Could you check a few things on this model? Use its own coordinates, in mm. A direction names the side the tool comes from. Give positions to 0.01 mm unless a question says otherwise; leave off trailing zeros. Write each loop counter-clockwise with the first axis right and the second up, starting at its lowest first coordinate (ties: lowest second). Pieces come first, ordered by that corner, then holes. Notation, with made-up numbers: M 50,47 L 94,47 A21 ccw 94,75 Z; hole C 23.25,-14.75 d3. An arc over 180 degrees is marked long. One line per item, written item: value.
```python
from build123d import *

# Parameters (mm, degrees)
F0_W     = 2
F0_H     = 7
F0_W_2   = 3
F0_H_2   = 12
F1_DEPTH = 7
F2_R     = 1.5
F3_DEPTH = 12
F4_R     = 3
F5_R     = 1.5
F6_DEPTH = 25
F7_R     = 1


with BuildPart() as f1:
    # F0 (on Top) → F1 (new body)
    with BuildSketch(Plane.XY):
        with Locations((-3, -4.5)):
            Rectangle(F0_W, F0_H)
        with Locations((-6, 7)):
            Rectangle(F0_W_2, F0_H_2)
        with Locations((6, 7)):
            Rectangle(F0_W_2, F0_H_2)
        Polygon((4, -1), (7.5, -1), (7.5, 1), (4.5, 1), (-4.5, 1), (-7.5, 1), (-7.5, -1), (-4, -1), (-2, -1), (2, -1), align=None)
        with Locations((3, -4.5)):
            Rectangle(F0_W, F0_H)
    extrude(amount=F1_DEPTH)

    # F2 (on face) → F3 (cut)
    with BuildSketch(Plane.YZ.offset(4)):
        with Locations((-4.5, 3.5)):
            Circle(F2_R)
    extrude(amount=-F3_DEPTH, mode=Mode.SUBTRACT)

    # F4
    f4_edges = [f1.edges().sort_by_distance(p)[0] for p in [
        (-3, -8, 0),
        (3, -8, 0),
        (3, -8, 7),
        (-3, -8, 7),
        (-6, 13, 0),
        (6, 13, 0),
        (-6, 13, 7),
        (6, 13, 7),
    ]]
    fillet(f4_edges, radius=F4_R)

    # F5 (on face) → F6 (cut)
    with BuildSketch(Plane(origin=(-7.5, 0, 0), x_dir=(0, -1, 0), z_dir=(-1, 0, 0))):
        with Locations((-9.5, 3.5)):
            Circle(F5_R)
    extrude(amount=-F6_DEPTH, mode=Mode.SUBTRACT)

    # F7
    f7_edges = [f1.edges().sort_by_distance(p)[0] for p in [
        (4.5, 11, 3.5),
        (-4.5, 11, 3.5),
    ]]
    fillet(f7_edges, radius=F7_R)


solid = f1.part
```
1) I'm going to push flat-ended pins straight in: pin 1 (1.8 mm diameter, centred on x = 5.5, z = 2, fed in from -Y); pin 2 (2 mm diameter, centred on x = 0.5, z = 4.5, fed in from +Y); pin 3 (3 mm diameter, centred on x = -5, z = 2, fed in from -Y); pin 4 (2 mm diameter, centred on y = -6, z = 4, fed in from +X). Where does each tip first touch, or does it pass through?
Outcome:
pin 1: stops at y = -1
pin 2: stops at y = 1
pin 3: stops at y = -8
pin 4: stops at x = 4
2) If we section it at A-A, the plane y = 5.25: Write out the boundary of the cut face in (x, z), then the cut area to 3 significant figures.
Outcome:
outline: M -7.5,0 L -4.5,0 L -4.5,7 L -7.5,7 Z; M 4.5,0 L 7.5,0 L 7.5,7 L 4.5,7 Z
area: 42.0 mm^2
3) If we section it at D-D, the plane z = 3.5: Give the number of separate pieces and of enclosed holes in the cut face, then the cut area to 3 significant figures.
Outcome:
separate pieces: 5
enclosed holes: 0
area: 99.1 mm^2
4) On a 3-axis mill with a long thin cutter (end or side, diameter ignored), from which of +Z, -Z, +X, -X, +Y, -Y can I reach the whole of each face in a straight line? I mean faces 5 (the face through (6, -1, 3)), 6 (the face through (3, -8, 3.5)), 7 (the face through (0, 1, 3)), 8 (the face through (-6, -1, 3)), 9 (the face through (2, -3, 4.2)). Say none if no direction works.
Outcome:
face 5: +Z, -Z, +X, -Y
face 6: +Z, -Z, +X, -X, -Y
face 7: +Z, -Z, +Y
face 8: +Z, -Z, -X, -Y
face 9: +Z, -Z, -Y
5) Please list where these lines run through material, in increasing order: L1, parallel to Z at x = -6.8, y = 9.5; L2, parallel to X at y = 4, z = 3; L3, parallel to Y at x = 5.5, z = 4.75. Write a range as from..to.
Outcome:
L1: z = 0..2, 5..7
L2: x = -7.5..-4.5, 4.5..7.5
L3: y = -1..8.67, 10.33..12.9
6) If we section it at C-C, the plane x = -6: Write out the boundary of the cut face in (y, z).
Outcome:
outline: M -1,0 L 10,0 A3 ccw 13,3 L 13,4 A3 ccw 10,7 L -1,7 Z; hole C 9.5,3.5 d3
7) If we section it at B-B, the plane y = 9.5: Write out the boundary of the cut face in (x, z), then the cut area to 3 significant figures.
Outcome:
outline: M -7.5,0 L -4.5,0 L -4.5,1 A1 ccw -5.5,2 L -7.5,2 Z; M -7.5,5 L -5.5,5 A1 ccw -4.5,6 L -4.5,7 L -7.5,7 Z; M 4.5,0 L 7.5,0 L 7.5,2 L 5.5,2 A1 ccw 4.5,1 Z; M 4.5,6 A1 ccw 5.5,5 L 7.5,5 L 7.5,7 L 4.5,7 Z
area: 23.1 mm^2
8) We'd pull the mould along X, two halves only. Please class faces 1 (the face through (-2, -3, 4.2)), 2 (the face through (-4, -3, 4.2)), 3 (the face through (6.02, 12.1, 6.14)), 4 (the face through (4.5, 6, 3)): pulls with the +X half, pulls with the -X half, needs draft (parallel to the pull), parting line crosses it, or undercut.
Outcome:
face 1: undercut
face 2: pulls with the -X half
face 3: needs draft
face 4: undercut
